Could you check a few things on this model? Use its own coordinates, in mm. A direction names the side the tool comes from. Give positions to 0.01 mm unless a question says otherwise; leave off trailing zeros. Order: outer loops, then holes, each group sorted by start corner. A loop starts at its lowest first (then second) coordinate and runs counter-clockwise, first axis right, second up. Notation, with made-up numbers: (42, 2.25) - (101, 2.25) arc R16 cw to (101, 25.25) - close; hole circle Ø8 at (-39, -6). An arc over 180 degrees is marked (long way). Put each result on its own line as item: value.
from build123d import *

# Parameters (mm, degrees)
BOSS_EXTRUDE1_DEPTH = 10
BOSS_EXTRUDE2_DEPTH = 12
CHAMFER2_SIZE       = 5.5
CHAMFER2_SIZE2      = 9
SKETCH6_W           = 14
SKETCH6_H           = 15
SKETCH6_W_2         = 17
SKETCH6_H_2         = 2.5
SKETCH6_W_3         = 1.5
LPATTERN3_COUNT     = 3
LPATTERN3_PITCH     = 45
SKETCH7_R           = 1.5
CUT_EXTRUDE1_DEPTH  = 10
LPATTERN4_COUNT     = 3
LPATTERN4_PITCH     = 45
LPATTERN5_COUNT     = 2
LPATTERN5_PITCH     = 45


with BuildPart() as part:
    # Sketch1 → Boss-Extrude1 (new body)
    with BuildSketch(Plane(origin=(0, 0, 0), x_dir=(1, 0, 0), z_dir=(0, 1, 0))):
        with BuildLine():
            Line((0, -11.4), (0, -31.5))
            Line((0, -31.5), (22, -31.5))
            Line((22, -31.5), (22, 121.5))
            Line((22, 121.5), (0, 121.5))
            Line((0, 121.5), (0, 101.4))
            ThreePointArc((0, 101.4), (11.4, 90), (0, 78.6))
            Line((0, 78.6), (0, 56.4))
            ThreePointArc((0, 56.4), (11.4, 45), (0, 33.6))
            Line((0, 33.6), (0, 11.4))
            ThreePointArc((0, 11.4), (11.4, 0), (0, -11.4))
        make_face()
    extrude(amount=-BOSS_EXTRUDE1_DEPTH)

    # Sketch3 → Boss-Extrude2 (add)
    with BuildSketch(Plane.XZ.offset(10)):
        with BuildLine():
            Line((0, -121.5), (0, -101.4))
            ThreePointArc((0, -101.4), (11.4, -90), (0, -78.6))
            Line((0, -78.6), (0, -56.4))
            ThreePointArc((0, -56.4), (11.4, -45), (0, -33.6))
            Line((0, -33.6), (0, -11.4))
            ThreePointArc((0, -11.4), (11.4, 0), (0, 11.4))
            Line((0, 11.4), (0, 31.5))
            Line((0, 31.5), (5, 31.5))
            Line((5, 31.5), (5, 15.619218931))
            ThreePointArc((5, 15.619218931), (16.4, 0), (5, -15.619218931))
            Line((5, -15.619218931), (5, -29.380781069))
            ThreePointArc((5, -29.380781069), (16.4, -45), (5, -60.619218931))
            Line((5, -60.619218931), (5, -74.380781069))
            ThreePointArc((5, -74.380781069), (16.4, -90), (5, -105.619218931))
            Line((5, -105.619218931), (5, -121.5))
            Line((5, -121.5), (0, -121.5))
        make_face()
    extrude(amount=BOSS_EXTRUDE2_DEPTH)

    # Chamfer2
    chamfer2_edges = [part.edges().sort_by_distance(p)[0] for p in [
        (22, -10, -45),
    ]]
    chamfer2_side = [part.faces().sort_by_distance(p)[0] for p in [
        (6.539415473, -10, 23.559609465),
    ]]
    chamfer(chamfer2_edges, length=CHAMFER2_SIZE, length2=CHAMFER2_SIZE2, reference=chamfer2_side[0])

    # Sketch6 → Cut-Revolve6 (revolve, cut)
    with BuildSketch(Plane.ZY):
        with Locations((-83, -18.5)):
            Rectangle(SKETCH6_W, SKETCH6_H)
        Polygon((-90, -11), (-76, -11), (-73, -8), (-73, -2.5), (-90, -2.5), align=None)
        with Locations((-81.5, -1.25)):
            Rectangle(SKETCH6_W_2, SKETCH6_H_2)
        with Locations((-72.25, -1.25)):
            Rectangle(SKETCH6_W_3, SKETCH6_H_2)
    cut_revolve6 = revolve(axis=Axis((0, 0, -90), (0, -1, 0)), mode=Mode.SUBTRACT)

    # LPattern3: Cut-Revolve6 ×3
    with Locations(*[(0, 0, i * LPATTERN3_PITCH) for i in range(1, LPATTERN3_COUNT)]):
        add(cut_revolve6, mode=Mode.SUBTRACT)

    # Sketch7 → Cut-Extrude1 (cut)
    with BuildSketch(Plane(origin=(5, 0, 0), x_dir=(0, 0, -1), z_dir=(1, 0, 0))):
        with Locations((67.5, -13)):
            Circle(SKETCH7_R)
    cut_extrude1 = extrude(amount=-CUT_EXTRUDE1_DEPTH, mode=Mode.SUBTRACT)

    # LPattern4: Cut-Extrude1 ×3
    with Locations(*[(0, 0, i * LPATTERN4_PITCH) for i in range(1, LPATTERN4_COUNT)]):
        add(cut_extrude1, mode=Mode.SUBTRACT)

    # LPattern5: Cut-Extrude1 ×2
    with Locations(*[(0, 0, -i * LPATTERN5_PITCH) for i in range(1, LPATTERN5_COUNT)]):
        add(cut_extrude1, mode=Mode.SUBTRACT)


solid = part.part
1) If I drill on line 1 (Z direction, x = 1, y = -8); line 2 (Z direction, x = 1, y = -2.25); line 3 (Y direction, x = 2.7, z = -22.5), over which ranges is the centre line in solid material (lowest first)? Write a range as [from, to].
Filled in:
line 1: z = [-121.5, -106.97], [-73.03, -61.97], [-28.03, -16.97], [16.97, 31.5]
line 2: z = [-121.5, -108.47], [-71.53, -63.47], [-26.53, -18.47], [18.47, 31.5]
line 3: y = [-22, -14.5], [-11.5, 0]
2) I'm going to push flat-ended pins straight in: pin 1 (10 mm diameter, centred on x = 12.5, y = -11, fed in from +Z); pin 2 (4 mm diameter, centred on y = -13, z = -67.5, fed in from +X); pin 3 (9 mm diameter, centred on x = 13, z = -21.5, fed in from -Y); pin 4 (5 mm diameter, centred on y = -7.5, z = -84.5, fed in from -X). Where does each tip first touch, or does it pass through?
Filled in:
pin 1: stops at z = 31.5
pin 2: stops at x = 5
pin 3: stops at y = -10
pin 4: stops at x = 13.75
3) We'd pull the mould along Z, two halves only. Please class faces 1 (the flat face through (5, -16, -113)), 2 (the cylindrical face through (18.496, -1.232, -45.407)): pulls with the +Z half, pulls with the -Z half, needs draft (parallel to the pull), parting line crosses it, or undercut.
Filled in:
face 1: needs draft
face 2: undercut
4) Suppose I cut it at B-B, the plane z = -112.5. List the corners of the cut face in (x, y) for me.
Filled in:
outline: (0, -22) - (5, -22) - (5, -14.5) - (0, -14.5) - close; (0, -11.5) - (5, -11.5) - (5, -10) - (16.5, -10) - (22, -1) - (22, 0) - (0, 0) - close
5) Suppose I cut it at C-C, the plane z = -45. List the corners of the cut face in (x, y) for me.
Filled in:
outline: (14, -22) - (16.4, -22) - (16.4, -10) - (16.5, -10) - (22, -1) - (22, 0) - (18.5, 0) - (18.5, -2.5) - (17, -2.5) - (17, -8) - (14, -11) - close
6) Which directions (+Z, -Z, +X, -X, +Y, -Y) give clear straight access to the entire face, cutting with the end or side of a thin tool? Please do faces 3 (the flat face through (12, -10, -29)), 4 (the cylindrical face through (17, -5, -45)), 5 (the flat face through (5, -16, 24)), 6 (the flat face through (0, -11, -113)).
Filled in:
face 3: +X, -Y
face 4: -X, +Y
face 5: +Z, +X, -Y
face 6: +Z, -Z, -X, +Y, -Y
7) Suppose I cut it at A-A, the plane y = -13. State how many separate pieces and enclosed holes the cut face has, and give its area (3 significant figures).
Filled in:
separate pieces: 5
enclosed holes: 0
area: 565 mm^2
